Geometry: final body of the model. Coordinates: model frame, mm. A direction names the side the tool comes from. Give positions to 0.01 mm unless a question says otherwise; leave off trailing zeros. Loops run counter-clockwise (first coordinate to the right, second up) from the corner with the lowest first, then second, coordinate; pieces in that order, holes last.
from build123d import *

# Parameters (mm, degrees)
F1_DEPTH = 4.7625
F2_R     = 5.08
F3_DEPTH = 3.175
F6_DEPTH = 15.875
F7_R     = 2.22249


# Not quite as in the source:
# - a fillet or chamfer is up to 0.001 mm smaller than in the source, because OpenCascade refuses the exact size


with BuildPart() as f1:
    # F0 (on Top) → F1 (new body)
    with BuildSketch(Plane.XY):
        with BuildLine():
            Line((0, 15.875), (0, 0))
            Line((0, 0), (4.7625, 0))
            Line((4.7625, 0), (4.7625, 2.6723581453))
            ThreePointArc((4.7625, 2.6723581453), (3.1538333333, 8.0077018914), (4.7625, 13.3430456375))
            Line((4.7625, 13.3430456375), (4.7625, 15.875))
            Line((4.7625, 15.875), (3.175, 15.875))
            Line((3.175, 15.875), (0, 15.875))
        make_face()
    extrude(amount=F1_DEPTH)


with BuildPart() as f1b:
    # F0 (on Top) → F1, piece 2 (new body)
    with BuildSketch(Plane.XY):
        with BuildLine():
            Line((20.6375, 2.3662392068), (20.6375, 0))
            Line((20.6375, 0), (25.4, 0))
            Line((25.4, 0), (25.4, 15.875))
            Line((25.4, 15.875), (20.8491666667, 15.875))
            Line((20.8491666667, 15.875), (20.8491666667, 13.3430456375))
            ThreePointArc((20.8491666667, 13.3430456375), (22.4560393469, 7.8216161703), (20.6375, 2.3662392068))
        make_face()
        with BuildLine():
            Line((25.4, 15.875), (25.4, 0))
            Line((25.4, 0), (30.1625, 0))
            Line((30.1625, 0), (30.1625, 2.3662392068))
            ThreePointArc((30.1625, 2.3662392068), (28.3439606531, 7.8216161703), (29.9508333333, 13.3430456375))
            Line((29.9508333333, 13.3430456375), (29.9508333333, 15.875))
            Line((29.9508333333, 15.875), (25.4, 15.875))
        make_face()
    extrude(amount=F1_DEPTH)


with BuildPart() as f1c:
    # F0 (on Top) → F1, piece 3 (new body)
    with BuildSketch(Plane.XY):
        with BuildLine():
            Line((46.0375, 2.6723581453), (46.0375, 0))
            Line((46.0375, 0), (50.8, 0))
            Line((50.8, 0), (50.8, 15.875))
            Line((50.8, 15.875), (46.0375, 15.875))
            Line((46.0375, 15.875), (46.0375, 13.3430456375))
            ThreePointArc((46.0375, 13.3430456375), (47.6461666667, 8.0077018914), (46.0375, 2.6723581453))
        make_face()
    extrude(amount=F1_DEPTH)


with BuildPart() as f3:
    # F2 (on face) → F3 (new body)
    with BuildSketch(Plane.XY.offset(4.7625)):
        with BuildLine():
            Line((25.4, 15.875), (4.7625, 15.875))
            Line((4.7625, 15.875), (4.7625, 13.3430456375))
            ThreePointArc((4.7625, 13.3430456375), (3.1538333333, 8.0077018914), (4.7625, 2.6723581453))
            Line((4.7625, 2.6723581453), (4.7625, 0))
            Line((4.7625, 0), (20.6375, 0))
            Line((20.6375, 0), (25.4, 0))
            Line((25.4, 0), (25.4, 2.2267585155))
            Line((25.4, 2.2267585155), (25.4, 15.875))
        make_face()
        with Locations((12.8058333333, 8.0077018914)):
            Circle(F2_R, mode=Mode.SUBTRACT)
        Polygon((46.0375, 15.875), (25.4, 15.875), (25.4, 2.2267585155), (25.4, 0), (30.1625, 0), (50.8, 0), (50.8, 15.875), align=None)
        with Locations((37.9941666667, 8.0077018914)):
            Circle(F2_R, mode=Mode.SUBTRACT)
        with BuildLine():
            Line((4.7625, 15.875), (0, 15.875))
            Line((0, 15.875), (0, 0))
            Line((0, 0), (4.7625, 0))
            Line((4.7625, 0), (4.7625, 2.6723581453))
            ThreePointArc((4.7625, 2.6723581453), (3.1538333333, 8.0077018914), (4.7625, 13.3430456375))
            Line((4.7625, 13.3430456375), (4.7625, 15.875))
        make_face()
    extrude(amount=F3_DEPTH)


with BuildPart() as f1_1:
    add(f1.part)

    # F4: union F3, F1b, F1c
    add(f3.part)
    add(f1b.part)
    add(f1c.part)

    # F5 (on face) → F6 (join)
    with BuildSketch(Plane.XZ):
        Polygon((56.6371664787, 20.0608457634), (44.5138207153, 7.9375), (50.8, 7.9375), (59.7802561211, 16.9177561211), align=None)
        Polygon((-8.9802561211, 16.9177561211), (0, 7.9375), (6.2861792847, 7.9375), (-5.8371664787, 20.0608457634), align=None)
    extrude(amount=-F6_DEPTH)

    # F7 (radius 2.2225 in the source; OpenCascade refuses exactly that, so slightly less here)
    f7_edges = [f1_1.edges().sort_by_distance(p)[0] for p in [
        (-8.980256, 7.9375, 16.917756),
        (-5.837166, 7.9375, 20.060846),
        (56.637166, 7.9375, 20.060846),
        (59.780256, 7.9375, 16.917756),
    ]]
    fillet(f7_edges, radius=F7_R)


solid = f1_1.part
Item 1: Set-up query: faces 1 (the face through (54.45, 7.83, 11.59)), 2 (the face through (1.084, 7.826, 13.14)), 3 (the face through (4.762, 15, 2)). Return all of +Z, -Z, +X, -X, +Y, -Y with unobstructed straight access to the full face (end or side cutting, diameter ignored); none if empty.
Values follow:
face 1: -Z, +X, +Y, -Y
face 2: +Z, +Y, -Y
face 3: -Z, +Y, -Y
Item 2: Section query C-C on x = 15.5. Return loops of the section in (y, z) (1 decimal).
Values follow:
outline: (0, 4.8) - (3.7, 4.8) - (3.7, 7.9) - (0, 7.9) - close; (12.3, 4.8) - (15.9, 4.8) - (15.9, 7.9) - (12.3, 7.9) - close
Item 3: Pin query (flat end, axial travel): pin 1 (2 mm diameter, centred on y = 14, z = 3, fed in from +X); pin 2 (1.5 mm diameter, centred on x = 29, y = 13, fed in from +Z); pin 3 (5 mm diameter, centred on x = 11, y = 10.5, fed in from -Z). Return the tip coordinate at first contact, or that it passes through.
Values follow:
pin 1: stops at x = 50.8
pin 2: stops at z = 7.94
pin 3: stops at z = 4.76
Item 4: Ray query, probe 1 along X at (y, z) = (15, 3.5); probe 2 along X at (y, z) = (6, 6.5); probe 3 along Z at (x, y) = (36, 14.75). Return the intervals inside material, ascending.
Values follow:
probe 1: x = 0 to 4.76, 20.85 to 29.95, 46.04 to 50.8
probe 2: x = 0 to 8.14, 17.47 to 33.33, 42.66 to 50.8
probe 3: z = 4.76 to 7.94
Item 5: Section query A-A on z = 2.5. Return loops of the section in (x, y) (1 decimal), plus the area to 3 significant figures.
Values follow:
outline: (0, 0) - (4.8, 0) - (4.8, 2.7) arc R9.7 cw to (4.8, 13.3) - (4.8, 15.9) - (0, 15.9) - close; (20.6, 0) - (30.2, 0) - (30.2, 2.4) arc R9.7 cw to (30, 13.3) - (30, 15.9) - (20.8, 15.9) - (20.8, 13.3) arc R9.7 cw to (20.6, 2.4) - close; (46, 0) - (50.8, 0) - (50.8, 15.9) - (46, 15.9) - (46, 13.3) arc R9.7 cw to (46, 2.7) - close
area: 250 mm2
Item 6: Draft query along X for faces 4 (the face through (2, 8, 0)), 5 (the face through (-8.06, 8.05, 16.94)), 6 (the face through (47.646, 8.087, 2.348)). Return one class per face: +X half, -X half, draft (parallel to the pull), parting line (faces both ways), or undercut.
Values follow:
face 4: draft
face 5: -X half
face 6: undercut
Item 7: Section query B-B on y = 5.75. Give the number of separate pieces and of enclosed holes in the cut face, plus the area to 3 significant figures.
Values follow:
separate pieces: 3
enclosed holes: 0
area: 295 mm2
